The model under review builds one solid part; all positions refer to its coordinate system, in mm. Face numbers are marked on the shaded views. A direction names the side the tool comes from. Coordinates: 2 decimals unless noted, no trailing zeros. Order: outer loops, then holes, each group sorted by start corner. A loop starts at its lowest first (then second) coordinate and runs counter-clockwise, first axis right, second up. Notation, with made-up numbers: M -11.75,72 L 41.25,72 A6 ccw 41.25,80 Z; hole C -34.75,46 d1. An arc over 180 degrees is marked long. Answer in a Markdown table with one row per item.
from build123d import *

# Parameters (mm, degrees)
SKETCH1_R           = 65
BOSS_EXTRUDE1_DEPTH = 5
SKETCH2_W           = 14
SKETCH2_H           = 70
BOSS_EXTRUDE2_DEPTH = 70
SKETCH4_W           = 41
SKETCH4_H           = 21
CUT_EXTRUDE1_DEPTH  = 12
CUT_EXTRUDE2_DEPTH  = 14
FILLET1_R           = 2
FILLET2_R           = 4
FILLET3_R           = 2
FILLET4_R           = 4
SKETCH7_R           = 1.3
CUT_EXTRUDE3_DEPTH  = 14
SKETCH8_W           = 20.5
SKETCH8_H           = 21
CUT_EXTRUDE4_DEPTH  = 2
SKETCH9_W           = 60
SKETCH9_H           = 4
BOSS_EXTRUDE3_DEPTH = 4
SKETCH10_R          = 2.5
SKETCH10_R_2        = 1.3
CUT_EXTRUDE5_DEPTH  = 3


with BuildPart() as part:
    # Sketch1 → Boss-Extrude1 (new body)
    with BuildSketch(Plane.XY):
        Circle(SKETCH1_R)
    extrude(amount=BOSS_EXTRUDE1_DEPTH)

    # Sketch2 → Boss-Extrude2 (add)
    with BuildSketch(Plane.XY.offset(5)):
        with Locations((-37, 0)):
            Rectangle(SKETCH2_W, SKETCH2_H)
        with Locations((37, 0)):
            Rectangle(SKETCH2_W, SKETCH2_H)
    extrude(amount=BOSS_EXTRUDE2_DEPTH)

    # Sketch4 → Cut-Extrude1 (cut)
    with BuildSketch(Plane.ZY.offset(44)):
        with Locations((35.5, 0)):
            Rectangle(SKETCH4_W, SKETCH4_H)
    cut_extrude1 = extrude(amount=-CUT_EXTRUDE1_DEPTH, mode=Mode.SUBTRACT)

    # Sketch5 → Cut-Extrude2 (cut)
    with BuildSketch(Plane.ZY.offset(44)):
        with BuildLine():
            Line((56, -21), (5, -21))
            Line((5, -21), (5, -35))
            Line((5, -35), (75, -35))
            Line((75, -35), (75, -8.94427191))
            ThreePointArc((75, -8.94427191), (71.261608982, -14.425092419), (66, -18.466185313))
            ThreePointArc((66, -18.466185313), (61.158008745, -20.356692899), (56, -21))
        make_face()
        with BuildLine():
            Line((5, 35), (5, 21))
            Line((5, 21), (56, 21))
            ThreePointArc((56, 21), (61.158008745, 20.356692899), (66, 18.466185313))
            ThreePointArc((66, 18.466185313), (71.261608982, 14.425092419), (75, 8.94427191))
            Line((75, 8.94427191), (75, 35))
            Line((75, 35), (5, 35))
        make_face()
        with BuildLine():
            ThreePointArc((75, 8.94427191), (71.261608982, 14.425092419), (66, 18.466185313))
            Line((66, 18.466185313), (66, -18.466185313))
            ThreePointArc((66, -18.466185313), (71.261608982, -14.425092419), (75, -8.94427191))
            Line((75, -8.94427191), (75, 8.94427191))
        make_face()
    cut_extrude2 = extrude(amount=-CUT_EXTRUDE2_DEPTH, mode=Mode.SUBTRACT)

    # Fillet1
    fillet1_edges = [part.edges().sort_by_distance(p)[0] for p in [
        (-30, -20.356692899, 61.158008745),
        (-44, -20.356692899, 61.158008745),
        (-37, -18.466185313, 66),
        (-30, 20.356692899, 61.158008745),
        (-44, 20.356692899, 61.158008745),
        (-30, -21, 30.5),
        (-44, -21, 30.5),
        (-44, 21, 30.5),
        (-44, 0, 66),
        (-30, 21, 30.5),
        (-30, 0, 66),
    ]]
    fillet(fillet1_edges, radius=FILLET1_R)

    # Fillet2
    fillet2_edges = [part.edges().sort_by_distance(p)[0] for p in [
        (-30, 0, 5),
        (-44, 0, 5),
        (-37, 21, 5),
        (-37, -21, 5),
        (-43.414213562, 20.414213562, 5),
        (-30.585786438, 20.414213562, 5),
        (-30.585786438, -20.414213562, 5),
        (-43.414213562, -20.414213562, 5),
    ]]
    fillet(fillet2_edges, radius=FILLET2_R)

    # Mirror2: Cut-Extrude1 across plane
    add(cut_extrude1.mirror(Plane(origin=(0, 0, 0), x_dir=(0, 0, 1), z_dir=(1, 0, 0))), mode=Mode.SUBTRACT)

    # Mirror3: Cut-Extrude2 across plane
    add(cut_extrude2.mirror(Plane(origin=(0, 0, 0), x_dir=(0, 0, 1), z_dir=(1, 0, 0))), mode=Mode.SUBTRACT)

    # Fillet3
    fillet3_edges = [part.edges().sort_by_distance(p)[0] for p in [
        (44, -20.356692899, 61.158008745),
        (44, 20.356692899, 61.158008745),
        (44, -21, 30.5),
        (30, 0, 66),
        (44, 0, 66),
        (30, 21, 30.5),
        (44, 21, 30.5),
        (30, -20.356692899, 61.158008745),
        (30, -21, 30.5),
        (30, 20.356692899, 61.158008745),
    ]]
    fillet(fillet3_edges, radius=FILLET3_R)

    # Fillet4
    fillet4_edges = [part.edges().sort_by_distance(p)[0] for p in [
        (30, 0, 5),
        (44, 0, 5),
        (37, 21, 5),
        (37, -21, 5),
        (30.585786438, 20.414213562, 5),
        (30.585786438, -20.414213562, 5),
        (43.414213562, 20.414213562, 5),
        (43.414213562, -20.414213562, 5),
    ]]
    fillet(fillet4_edges, radius=FILLET4_R)

    # Sketch7 → Cut-Extrude3 (cut)
    with BuildSketch(Plane.ZY.offset(44)):
        with Locations((59.5, 5)):
            Circle(SKETCH7_R)
        with Locations((59.5, -5)):
            Circle(SKETCH7_R)
        with Locations((11.5, -5)):
            Circle(SKETCH7_R)
        with Locations((11.5, 5)):
            Circle(SKETCH7_R)
    cut_extrude3 = extrude(amount=-CUT_EXTRUDE3_DEPTH, mode=Mode.SUBTRACT)

    # Mirror6: Cut-Extrude3 across plane
    add(cut_extrude3.mirror(Plane(origin=(0, 0, 0), x_dir=(0, 0, 1), z_dir=(1, 0, 0))), mode=Mode.SUBTRACT)

    # Sketch8 → Cut-Extrude4 (cut)
    with BuildSketch(Plane.ZY.offset(32)):
        with Locations((45.75, 0)):
            Rectangle(SKETCH8_W, SKETCH8_H)
    cut_extrude4 = extrude(amount=-CUT_EXTRUDE4_DEPTH, mode=Mode.SUBTRACT)

    # Mirror7: Cut-Extrude4 across plane
    add(cut_extrude4.mirror(Plane(origin=(0, 0, 0), x_dir=(0, 0, 1), z_dir=(1, 0, 0))), mode=Mode.SUBTRACT)

    # Sketch9 → Boss-Extrude3 (add)
    with BuildSketch(Plane.XY.offset(30)):
        with Locations((0, -17)):
            Rectangle(SKETCH9_W, SKETCH9_H)
    boss_extrude3 = extrude(amount=-BOSS_EXTRUDE3_DEPTH)

    # Mirror8: Boss-Extrude3 across plane
    add(boss_extrude3.mirror(Plane.ZX))

    # Sketch10 → Cut-Extrude5 (cut)
    with BuildSketch(Plane(origin=(-30, 0, 0), x_dir=(0, 0, -1), z_dir=(1, 0, 0))):
        with Locations((-59.5, 5)):
            Circle(SKETCH10_R)
        with Locations((-59.5, 5)):
            Circle(SKETCH10_R_2, mode=Mode.SUBTRACT)
        with Locations((-59.5, -5)):
            Circle(SKETCH10_R)
        with Locations((-59.5, -5)):
            Circle(SKETCH10_R_2, mode=Mode.SUBTRACT)
    cut_extrude5 = extrude(amount=-CUT_EXTRUDE5_DEPTH, mode=Mode.SUBTRACT)

    # Mirror9: Cut-Extrude5 across plane
    add(cut_extrude5.mirror(Plane(origin=(0, 0, 0), x_dir=(0, 0, 1), z_dir=(1, 0, 0))), mode=Mode.SUBTRACT)


solid = part.part
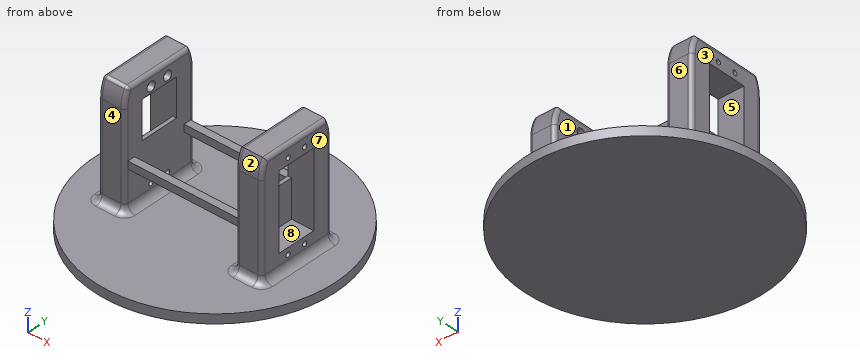
(1) To check wall thickness, follow line 1 (X direction, y = 17, z = 47); line 2 (Y direction, x = 28, z = 26.5); line 3 (Y direction, x = -40, z = 11). State the ranges of each line that lie inside material, in increasing order. Write a range as [from, to].
Report:
| item | result |
|---|---|
| line 1 | [-44, -30], [30, 44] |
| line 2 | [-19, -15], [15, 19] |
| line 3 | [-21, -6.2], [-3.8, 3.8], [6.2, 21] |
(2) Take a section at B-B (y = 0). State how many separate pieces and enclosed holes the cut face has, then the cut area to 3 significant figures.
Report:
| item | result |
|---|---|
| separate pieces | 3 |
| enclosed holes | 0 |
| area | 1,300 mm^2 |
(3) Take a section at D-D (y = -13). Write out the cut boundary in (x, z), then the cut area to 3 significant figures.
Report:
| item | result |
|---|---|
| outline | M -63.69,0 L 63.69,0 L 63.69,5 L 48,5 A4 cw 44,9 L 44,64 A2 ccw 42,66 L 32,66 A2 ccw 30,64 L 30,9 A4 cw 26,5 L -26,5 A4 cw -30,9 L -30,64 A2 ccw -32,66 L -42,66 A2 ccw -44,64 L -44,9 A4 cw -48,5 L -63.69,5 Z |
| area | 2,360 mm^2 |
(4) Take a section at C-C (z = 42.5). Write out the cut boundary in (x, y).
Report:
| item | result |
|---|---|
| outline | M -44,-19 A2 ccw -42,-21 L -32,-21 A2 ccw -30,-19 L -30,-10.5 L -44,-10.5 Z; M -44,10.5 L -30,10.5 L -30,19 A2 ccw -32,21 L -42,21 A2 ccw -44,19 Z; M 30,-19 A2 ccw 32,-21 L 42,-21 A2 ccw 44,-19 L 44,-10.5 L 30,-10.5 Z; M 30,10.5 L 44,10.5 L 44,19 A2 ccw 42,21 L 32,21 A2 ccw 30,19 Z |
(5) Insertion check: P1, Ø1, axis at x = 31, y = -1, coming from the +Z side; P2, Ø3, axis at x = 38.5, z = 33.5, coming from the +Y side; P3, Ø6, axis at x = -47.5, z = 35, coming from the +Y side; P4, Ø5.5, axis at y = -5, z = 58.5, coming from the -X side. Each pin has a flat end and moves straight along its axis. Give the tip position at first contact, or say it passes through.
Report:
| item | result |
|---|---|
| P1 | z = 65.94 |
| P2 | y = 21 |
| P3 | through |
| P4 | x = -44 |
(6) Machinability: for the marked faces 4, 5, 6, 7 and 8, which of the approach directions +Z, -Z, +X, -X, +Y, -Y give a long, thin tool a straight path to every point of the face, cutting with its end or side? Answer none if there is none.
Report:
| item | result |
|---|---|
| face 4 | +Z, +X, -X, -Y |
| face 5 | -X |
| face 6 | +Z, +X, -X, +Y |
| face 7 | +Z, +X, +Y, -Y |
| face 8 | +X |
(7) Take a section at A-A (x = 0). Write out the cut boundary in (y, z), then the cut area to 3 significant figures.
Report:
| item | result |
|---|---|
| outline | M -65,0 L 65,0 L 65,5 L -65,5 Z; M -19,26 L -15,26 L -15,30 L -19,30 Z; M 15,26 L 19,26 L 19,30 L 15,30 Z |
| area | 682 mm^2 |
(8) The part is to be moulded in two halves that separate along X. For the marked faces 1, 2 and 3, say which applies: +X half, -X half, draft (parallel to the pull), parting line (faces both ways), or undercut.
Report:
| item | result |
|---|---|
| face 1 | undercut |
| face 2 | draft |
| face 3 | -X half |
